Build history of the part. All positions in model axes, mm. Face numbers are marked on the shaded views. A direction names the side the tool comes from. Give positions to 0.01 mm unless a question says otherwise; leave off trailing zeros. Order: outer loops, then holes, each group sorted by start corner. A loop starts at its lowest first (then second) coordinate and runs counter-clockwise, first axis right, second up. Notation, with made-up numbers: (-34.5, 58) -> (15.5, 58) arc R5 cw to (15.5, 65) -> close; hole circle Ø8 at (24.25, 35.25). An arc over 180 degrees is marked (long way). Use a Markdown table: item, result. Add a question column.
```python
from build123d import *

# Parameters (mm, degrees)
F0_W        = 101.6
F0_H        = 152.4
F4_DEPTH    = 12.7
F1_R        = 29.21
F2_R        = 4.426371
F2_W        = 25.4
F2_H        = 12.7
F3_R        = 3.556
F5_DEPTH    = 25.4
F5_FACE_W   = 25.4
F5_FACE_H   = 12.7
F5_FACE_R   = 29.21
F5_FACE_R_2 = 3.556
F5_FACE_R_3 = 4.426371
F6_DEPTH    = 25.4


with BuildPart() as f4:
    # F0 (on Top) → F4 (new body)
    with BuildSketch(Plane.XY):
        with Locations((-86.551244, 14.376812)):
            Rectangle(F0_W, F0_H)
    extrude(amount=F4_DEPTH)

    # F1 (on Top) + F2 (on Top) + F3 (on Top) → F5 (join)
    with BuildSketch(Plane.XY):
        with Locations((-81.815682, 41.263096)):
            Circle(F1_R)
    with BuildSketch(Plane.XY):
        with Locations((-119.990457, -26.553331)):
            Circle(F2_R)
        with Locations((-81.890457, -29.590288)):
            Rectangle(F2_W, F2_H)
    with BuildSketch(Plane.XY):
        with Locations((-51.804963, -10.494831)):
            Circle(F3_R)
        with Locations((-51.804963, -35.894831)):
            Circle(F3_R)
    extrude(amount=F5_DEPTH)

    # F5_face (on face) → F6 (cut)
    with BuildSketch(Plane(origin=(-81.890457, -29.590288, 25.4), x_dir=(1, 0, 0), z_dir=(0, 0, 1))):
        Rectangle(F5_FACE_W, F5_FACE_H)
        with Locations((0.074775, 70.853384)):
            Circle(F5_FACE_R)
        with Locations((30.085494, 19.095457)):
            Circle(F5_FACE_R_2)
        with Locations((30.085494, -6.304543)):
            Circle(F5_FACE_R_2)
        with Locations((-38.1, 3.036957)):
            Circle(F5_FACE_R_3)
    extrude(amount=-F6_DEPTH, mode=Mode.SUBTRACT)


solid = f4.part
```
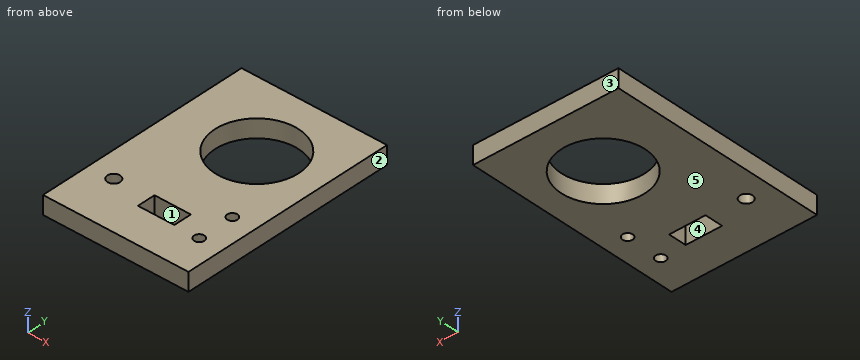
(1) Band-saw the part on A-A on y = 46. Give the cut face in (x, z), plus the area to 3 significant figures.
(2) Tool access for the marked faces 4 and 5: list every direction of +Z, -Z, +X, -X, +Y, -Y with a clear straight run to the whole face (end or side of a thin tool).
(3) Mould opens along X. For the marked faces 1, 2 and 3 say: released by +X, released by -X, zero draft, split by the parting line, or undercut.
(4) Wall check: probe 1 along Y at (x, z) = (-87, 5.5); probe 2 along Y at (x, z) = (-64, 11); probe 3 along Y at (x, z) = (-60, 9.25). Give the ranges that are in metal, low to high.
(5) Band-saw the part on C-C on z = 2. Give the cut face in (x, y), plus the area to 3 significant figures.
(6) Band-saw the part on B-B on x = -66. Give the cut face in (y, z).
Response:
| question | item | result |
|---|---|---|
| 1 | outline | (-137.35, 0) -> (-110.64, 0) -> (-110.64, 12.7) -> (-137.35, 12.7) -> close; (-52.99, 0) -> (-35.75, 0) -> (-35.75, 12.7) -> (-52.99, 12.7) -> close |
| 1 | area | 558 mm² |
| 2 | face 4 | +Z, -Z |
| 2 | face 5 | -Z, +X, -X, +Y, -Y |
| 3 | face 1 | undercut |
| 3 | face 2 | released by +X |
| 3 | face 3 | zero draft |
| 4 | probe 1 | y = -61.82 to -35.94, -23.24 to 12.52, 70.01 to 90.58 |
| 4 | probe 2 | y = -61.82 to 18.12, 64.41 to 90.58 |
| 4 | probe 3 | y = -61.82 to 21.84, 60.69 to 90.58 |
| 5 | outline | (-137.35, -61.82) -> (-35.75, -61.82) -> (-35.75, 90.58) -> (-137.35, 90.58) -> close; hole circle Ø8.85 at (-119.99, -26.55); hole circle Ø58.42 at (-81.82, 41.26); hole (-94.59, -35.94) -> (-69.19, -35.94) -> (-69.19, -23.24) -> (-94.59, -23.24) -> close; hole circle Ø7.11 at (-51.8, -35.89); hole circle Ø7.11 at (-51.8, -10.49) |
| 5 | area | 12,300 mm² |
| 6 | outline | (-61.82, 0) -> (16.71, 0) -> (16.71, 12.7) -> (-61.82, 12.7) -> close; (65.82, 0) -> (90.58, 0) -> (90.58, 12.7) -> (65.82, 12.7) -> close |
